```python
from build123d import *

# Parameters (mm, degrees)
SKETCH1_W           = 121
SKETCH1_H           = 78
BOSS_EXTRUDE3_DEPTH = 35
SKETCH4_W           = 117
SKETCH4_H           = 74
CUT_EXTRUDE1_DEPTH  = 33
SKETCH5_W           = 10
SKETCH5_H           = 23
SKETCH5_W_2         = 13
SKETCH5_H_2         = 24
CUT_EXTRUDE2_DEPTH  = 33
SKETCH6_R           = 3
CUT_EXTRUDE3_DEPTH  = 33
CUT_EXTRUDE4_DEPTH  = 1


with BuildPart() as part:
    # Sketch1 → Boss-Extrude3 (new body)
    with BuildSketch(Plane(origin=(0, 0, 0), x_dir=(1, 0, 0), z_dir=(0, 1, 0))):
        with Locations((60.5, 39)):
            Rectangle(SKETCH1_W, SKETCH1_H)
    extrude(amount=BOSS_EXTRUDE3_DEPTH)

    # Sketch4 → Cut-Extrude1 (cut)
    with BuildSketch(Plane(origin=(0, 35, 0), x_dir=(1, 0, 0), z_dir=(0, 1, 0))):
        with Locations((60.5, 39)):
            Rectangle(SKETCH4_W, SKETCH4_H)
    extrude(amount=-CUT_EXTRUDE1_DEPTH, mode=Mode.SUBTRACT)

    # Sketch5 → Cut-Extrude2 (cut)
    with BuildSketch(Plane(origin=(0, 0, -78), x_dir=(-1, 0, 0), z_dir=(0, 0, -1))):
        with Locations((-108, 23.5)):
            Rectangle(SKETCH5_W, SKETCH5_H)
        with Locations((-77.5, 23)):
            Rectangle(SKETCH5_W_2, SKETCH5_H_2)
    extrude(amount=-CUT_EXTRUDE2_DEPTH, mode=Mode.SUBTRACT)

    # Sketch6 → Cut-Extrude3 (cut)
    with BuildSketch(Plane(origin=(0, 0, -78), x_dir=(-1, 0, 0), z_dir=(0, 0, -1))):
        with Locations((-51, 9.463298595)):
            Circle(SKETCH6_R)
    extrude(amount=-CUT_EXTRUDE3_DEPTH, mode=Mode.SUBTRACT)

    # Sketch7 → Cut-Extrude4 (cut)
    with BuildSketch(Plane(origin=(0, 0, 0), x_dir=(-1, 0, 0), z_dir=(0, -1, 0))):
        with BuildLine():
            Line((-114.434159313, 75.289773702), (-114.434159313, 74.964132677))
            Line((-114.434159313, 74.964132677), (-115.514117246, 74.964132677))
            Line((-115.514117246, 74.964132677), (-115.685205988, 74.129041531))
            add(Edge.make_bspline(
                [(-115.685205988, 74.129041531), (-115.651591016, 74.138321849), (-115.586467325, 74.156300997), (-115.490346594, 74.176263375), (-115.399095095, 74.188297028), (-115.339881009, 74.189940145), (-115.311227623, 74.190735241)],
                knots=[0, 0, 0, 0, 0.000104595, 0.000202637, 0.000294305, 0.000380252, 0.000380252, 0.000380252, 0.000380252], degree=3))
            add(Edge.make_bspline(
                [(-115.311227623, 74.190735241), (-115.275773087, 74.189967856), (-115.206060613, 74.188458987), (-115.104062425, 74.173970238), (-115.006696157, 74.151164744), (-114.914165436, 74.119305413), (-114.826299079, 74.078565869), (-114.743905506, 74.027675209), (-114.66574797, 73.968227116), (-114.593228617, 73.899878427), (-114.527438709, 73.824656674), (-114.469593847, 73.743777748), (-114.42046064, 73.658027655), (-114.380944812, 73.566587103), (-114.349390452, 73.470467013), (-114.328388285, 73.368656028), (-114.314403128, 73.262113805), (-114.312840677, 73.189266088), (-114.312043929, 73.152118454)],
                knots=[0, 0, 0, 0, 0.000106308, 0.000209029, 0.000308378, 0.000405929, 0.000502102, 0.000598312, 0.00069588, 0.000796219, 0.000896736, 0.000995218, 0.001094066, 0.001192613, 0.001293582, 0.001396995, 0.001504047, 0.001615439, 0.001615439, 0.001615439, 0.001615439], degree=3))
            add(Edge.make_bspline(
                [(-114.312043929, 73.152118454), (-114.312647247, 73.126244726), (-114.31384573, 73.07484693), (-114.319940449, 72.998516119), (-114.331674991, 72.923801263), (-114.347429998, 72.850692451), (-114.367879192, 72.779328092), (-114.392634262, 72.70950392), (-114.42292923, 72.641654527), (-114.45615912, 72.575137918), (-114.493575568, 72.511457844), (-114.535103214, 72.451904835), (-114.578977624, 72.395585522), (-114.626186595, 72.343103922), (-114.677168926, 72.294804898), (-114.731307182, 72.250401814), (-114.788169363, 72.20914375), (-114.84863519, 72.172705459), (-114.911357299, 72.139174777), (-114.977241468, 72.111666997), (-115.04478796, 72.087073875), (-115.114968955, 72.067470947), (-115.187625485, 72.052110701), (-115.262877317, 72.041678013), (-115.340329782, 72.034079388), (-115.392830686, 72.033603721), (-115.419350619, 72.033363446)],
                knots=[0, 0, 0, 0, 7.7636e-05, 0.000154223, 0.000229512, 0.000304362, 0.000378447, 0.000452077, 0.000526407, 0.000601214, 0.00067506, 0.000747747, 0.00081887, 0.000889121, 0.000959302, 0.001029336, 0.001099058, 0.00116985, 0.001240974, 0.00131221, 0.00138383, 0.001456517, 0.001530612, 0.001606437, 0.001684346, 0.001763871, 0.001763871, 0.001763871, 0.001763871], degree=3))
            add(Edge.make_bspline(
                [(-115.419350619, 72.033363446), (-115.450986483, 72.033990135), (-115.513226308, 72.035223071), (-115.604412823, 72.048121268), (-115.692146786, 72.066594249), (-115.77572195, 72.094385723), (-115.85588731, 72.129208483), (-115.931563633, 72.173219581), (-116.004684587, 72.223093483), (-116.072277649, 72.281949231), (-116.135012123, 72.346279886), (-116.19117017, 72.41609146), (-116.241184201, 72.49023174), (-116.2842533, 72.56906078), (-116.320990791, 72.652371447), (-116.34985153, 72.740475884), (-116.373145466, 72.832913744), (-116.38300014, 72.896553), (-116.388005467, 72.928876267)],
                knots=[0, 0, 0, 0, 9.4843e-05, 0.000186593, 0.000275792, 0.000363484, 0.000450342, 0.000537514, 0.000625728, 0.000715478, 0.000805885, 0.000894984, 0.00098389, 0.001073836, 0.001164117, 0.001256635, 0.001351658, 0.001449737, 0.001449737, 0.001449737, 0.001449737], degree=3))
            Line((-116.388005467, 72.928876267), (-116.10306957, 72.928876267))
            add(Edge.make_bspline(
                [(-116.10306957, 72.928876267), (-116.096058664, 72.898599056), (-116.082583314, 72.840404576), (-116.053005242, 72.758642574), (-116.016841198, 72.685781564), (-115.973838682, 72.620857728), (-115.922539726, 72.564243852), (-115.864002315, 72.513791231), (-115.798372595, 72.468275221), (-115.725444451, 72.430335996), (-115.648506872, 72.397979342), (-115.567982331, 72.376433161), (-115.486063388, 72.361283065), (-115.430656581, 72.35976654), (-115.402814161, 72.359004472)],
                knots=[0, 0, 0, 0, 9.3172e-05, 0.000179081, 0.000260145, 0.000336703, 0.000411917, 0.000488562, 0.000568128, 0.000650923, 0.00073478, 0.000817953, 0.000900557, 0.000983994, 0.000983994, 0.000983994, 0.000983994], degree=3))
            add(Edge.make_bspline(
                [(-115.402814161, 72.359004472), (-115.375637572, 72.359749034), (-115.322126646, 72.361215085), (-115.243376317, 72.372499046), (-115.167346067, 72.3898777), (-115.094786107, 72.415885354), (-115.024426711, 72.447494491), (-114.958047648, 72.488057453), (-114.893728609, 72.534739041), (-114.833468802, 72.588221127), (-114.77827873, 72.647157921), (-114.729514249, 72.710183842), (-114.688895192, 72.77741841), (-114.654664965, 72.847697628), (-114.628672329, 72.921791747), (-114.610129439, 72.999353528), (-114.59924095, 73.080574545), (-114.597743094, 73.135973134), (-114.596979826, 73.164202789)],
                knots=[0, 0, 0, 0, 8.15e-05, 0.000160473, 0.000238226, 0.000315066, 0.000391338, 0.000469218, 0.000547964, 0.000629516, 0.000710512, 0.000789892, 0.000868102, 0.000945761, 0.001024012, 0.00110315, 0.001184644, 0.001269321, 0.001269321, 0.001269321, 0.001269321], degree=3))
            add(Edge.make_bspline(
                [(-114.596979826, 73.164202789), (-114.597577161, 73.189671506), (-114.598746359, 73.239522897), (-114.608299091, 73.312456463), (-114.624915201, 73.38146558), (-114.647978293, 73.446883492), (-114.677260417, 73.508771901), (-114.713043858, 73.567194677), (-114.756000155, 73.621381797), (-114.805069225, 73.671358613), (-114.858824733, 73.717482178), (-114.918191557, 73.756801457), (-114.981927348, 73.789879439), (-115.049264199, 73.818425409), (-115.121803785, 73.838927514), (-115.198109588, 73.85431981), (-115.279005601, 73.863223746), (-115.334314725, 73.864459174), (-115.36274505, 73.865094215)],
                knots=[0, 0, 0, 0, 7.6388e-05, 0.000149519, 0.000220172, 0.000288967, 0.000357247, 0.000425206, 0.000494043, 0.000564207, 0.000635056, 0.000706145, 0.000777268, 0.000850264, 0.000925136, 0.001002969, 0.001083601, 0.001168886, 0.001168886, 0.001168886, 0.001168886], degree=3))
            add(Edge.make_bspline(
                [(-115.36274505, 73.865094215), (-115.387354864, 73.864567536), (-115.438167887, 73.863480077), (-115.516112165, 73.855473184), (-115.598019657, 73.84255611), (-115.683576378, 73.824788585), (-115.773039267, 73.801537537), (-115.866219531, 73.773675097), (-115.963313087, 73.740362998), (-116.028734165, 73.715205919), (-116.062364441, 73.702273702)],
                knots=[0, 0, 0, 0, 7.3822e-05, 0.000152423, 0.000234822, 0.000322511, 0.00041445, 0.000512043, 0.000614219, 0.000722306, 0.000722306, 0.000722306, 0.000722306], degree=3))
            Line((-116.062364441, 73.702273702), (-115.736723416, 75.289773702))
            Line((-115.736723416, 75.289773702), (-114.434159313, 75.289773702))
        make_face()
        Polygon((-112.253254866, 75.371183959), (-112.195377262, 75.371183959), (-112.195377262, 73.173107036), (-111.829031108, 73.173107036), (-111.829031108, 72.84746601), (-112.195377262, 72.84746601), (-112.195377262, 72.114773702), (-112.480313159, 72.114773702), (-112.480313159, 72.84746601), (-113.986402903, 72.84746601), align=None)
        Polygon((-112.480313159, 73.173107036), (-112.480313159, 74.551993254), (-113.42670739, 73.173107036), align=None, mode=Mode.SUBTRACT)
    extrude(amount=-CUT_EXTRUDE4_DEPTH, mode=Mode.SUBTRACT)


solid = part.part
```
Geometry: final body of the model. Coordinates: model frame, mm. A direction names the side the tool comes from. Coordinates: 2 decimals unless noted, no trailing zeros. Write each loop counter-clockwise with the first axis right and the second up, starting at its lowest first coordinate (ties: lowest second). Pieces come first, ordered by that corner, then holes. Notation, with made-up numbers: M -27.5,-36.75 L -21.5,-36.75 A21 cw -21.5,-25.75 Z; hole C 14.25,75 d3. An arc over 180 degrees is marked long. Answer as CSV lines item,"result". Start each with the question number.
Q1. Pin query (flat end, axial travel): P1, Ø0.6, axis at x = 79.5, z = -76.5, coming from the +Y side; P2, Ø10, axis at y = 25.5, z = -34.5, coming from the -X side; P3, Ø6, axis at x = 75.5, z = -59, coming from the +Y side. Return the tip coordinate at first contact, or that it passes through.
Q2. Cut plane B-B on z = -17.5. Return the cut outline in (x, y).
Q3. Cut plane A-A on y = 26. Return the cut outline in (x, z).
Q4. Mould query, pull axis Y, two halves, no side actions, for faces 3 (the cylindrical face through (53.38, 7.64, -77.01)), 4 (the flat face through (60, 17, -78)), 5 (the flat face through (60, 2, -40)). Classes: released by +Y, released by -Y, zero draft, split by the parting line, or undercut.
Q5. Cut plane C-C on x = 99. Return the cut outline in (y, z), then the cut area to 3 significant figures.
Q6. Cut plane D-D on x = 51. Return the cut outline in (y, z).
Q7. Line query: line 1 (Z direction, x = 35.5, y = 6.5); line 2 (Y direction, x = 51, z = -76.95); line 3 (X direction, y = 14, z = -39). Output: solid intervals per line, ascending. Write a range as from..to.
Q8. Reachability of faces 1 (the flat face through (60, 17, 0)), 2 (the flat face through (119, 19, -38)) from +Z, -Z, +X, -X, +Y, -Y: full face, straight path, thin tool, end or side. Return the list, or none.
Findings below:
1,P1,"stops at y = 11"
1,P2,"stops at x = 0"
1,P3,"stops at y = 2"
2,outline,"M 0,0 L 121,0 L 121,35 L 119,35 L 119,2 L 2,2 L 2,35 L 0,35 Z"
3,outline,"M 0,-78 L 71,-78 L 71,-76 L 2,-76 L 2,-2 L 119,-2 L 119,-76 L 113,-76 L 113,-78 L 121,-78 L 121,0 L 0,0 Z; M 84,-78 L 103,-78 L 103,-76 L 84,-76 Z"
4,face 3,"undercut"
4,face 4,"zero draft"
4,face 5,"released by +Y"
5,outline,"M 0,-78 L 35,-78 L 35,-76 L 2,-76 L 2,-2 L 35,-2 L 35,0 L 0,0 Z"
5,area,"288 mm2"
6,outline,"M 0,-78 L 6.46,-78 L 6.46,-76 L 2,-76 L 2,-2 L 35,-2 L 35,0 L 0,0 Z; M 12.46,-78 L 35,-78 L 35,-76 L 12.46,-76 Z"
7,line 1,"z = -78..-76, -2..0"
7,line 2,"y = 0..6.46, 12.46..35"
7,line 3,"x = 0..2, 119..121"
8,face 1,"+Z, +X, -X, +Y, -Y"
8,face 2,"+Y"
